The figure shows three views and two pictorial views of one solid part (mm, origin at its lowest corner). Answer the questions. Give positions to 0.01 mm unless a question says otherwise; leave off trailing zeros. Order: outer loops, then holes, each group sorted by start corner. A loop starts at its lowest first (then second) coordinate and runs counter-clockwise, first axis right, second up. Notation, with made-up numbers: (-21, 70.25) -> (-3, 70.25) arc R31 ccw to (-3, 95.25) -> close; hole circle Ø8 at (-21.75, -18). An arc over 180 degrees is marked (long way). Use one line per item in the form item = value.
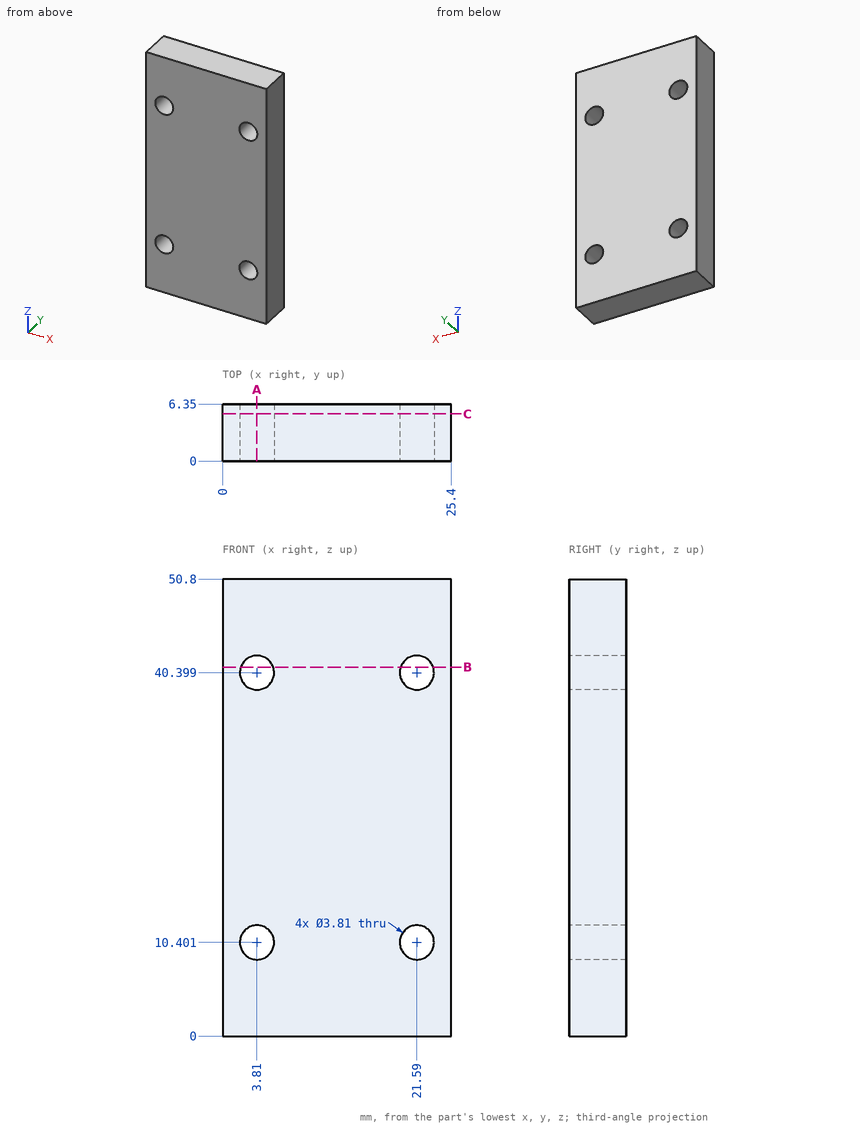
Item 1: The part is cut by section C-C on y = 5.25. Give the vertices of the cut face in (x, z) (1 decimal).
Checks:
outline = (0, 0) -> (25.4, 0) -> (25.4, 50.8) -> (0, 50.8) -> close; hole circle Ø3.8 at (3.8, 10.4); hole circle Ø3.8 at (3.8, 40.4); hole circle Ø3.8 at (21.6, 10.4); hole circle Ø3.8 at (21.6, 40.4)
Item 2: The part is cut by section A-A on x = 3.81. Give the vertices of the cut face in (y, z).
Checks:
outline = (0, 0) -> (6.35, 0) -> (6.35, 8.5) -> (0, 8.5) -> close; (0, 12.31) -> (6.35, 12.31) -> (6.35, 38.49) -> (0, 38.49) -> close; (0, 42.3) -> (6.35, 42.3) -> (6.35, 50.8) -> (0, 50.8) -> close
Item 3: The part is cut by section B-B on z = 41. Give the vertices of the cut face in (x, y).
Checks:
outline = (0, 0) -> (2, 0) -> (2, 6.35) -> (0, 6.35) -> close; (5.62, 0) -> (19.78, 0) -> (19.78, 6.35) -> (5.62, 6.35) -> close; (23.4, 0) -> (25.4, 0) -> (25.4, 6.35) -> (23.4, 6.35) -> close
Item 4: Straight lines are drawn through the part: L1, parallel to Z at x = 3.81, y = 4.5; L2, parallel to Z at x = 20.5, y = 4.25 (1 decimal); L3, parallel to X at y = 3.75, z = 39 (1 decimal). For each, find the intervals that lie inside material, in ascending order. Write a range as from..to.
Checks:
L1 = 0..8.5, 12.31..38.49, 42.3..50.8
L2 = 0..8.8, 12..38.8, 42..50.8
L3 = 0..2.5, 5.1..20.3, 22.9..25.4
